Read the model definition and answer for the solid it produces. Units are mm, in the model's axes. Face numbers are marked on the shaded views. A direction names the side the tool comes from. Give positions to 0.01 mm unless a question says otherwise; leave off trailing zeros. Order: outer loops, then holes, each group sorted by start corner. A loop starts at its lowest first (then second) coordinate and runs counter-clockwise, first axis right, second up.
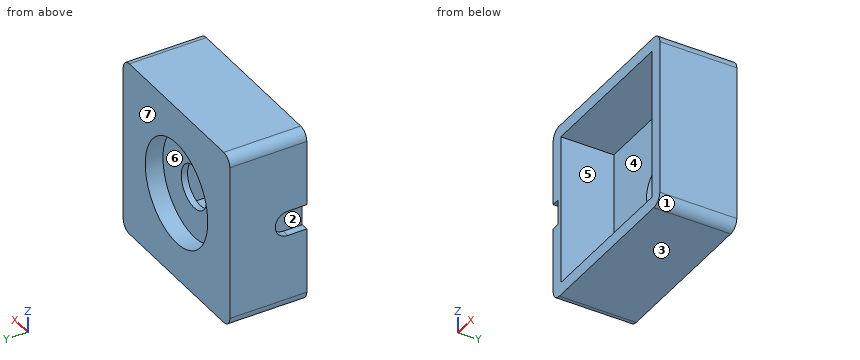
```python
from build123d import *

# Parameters (mm, degrees)
SKETCH_1_W          = 140
SKETCH_1_H          = 140
SKETCH_1_R          = 41
EXTRUDE_1_DEPTH     = 14
SKETCH_3_W          = 140
SKETCH_3_H          = 140
SKETCH_3_R          = 17
EXTRUDE_2_DEPTH     = 5
SKETCH_4_W          = 140
SKETCH_4_H          = 140
SKETCH_4_W_2        = 120
SKETCH_4_H_2        = 120
EXTRUDE_3_DEPTH     = 42
FILLET_3_R          = 8
CUT_EXTRUDE_1_DEPTH = 6


with BuildPart() as part:
    # 草图1 → 凸台-拉伸1 (new body)
    with BuildSketch(Plane(origin=(0, 0, 0), x_dir=(1, 0, 0), z_dir=(0, 1, 0))):
        Rectangle(SKETCH_1_W, SKETCH_1_H)
        with Locations(Location((0, 0, 0), (0, 0, 270))):
            Circle(SKETCH_1_R, mode=Mode.SUBTRACT)
    extrude(amount=EXTRUDE_1_DEPTH)

    # 草图3 → 凸台-拉伸2 (add)
    with BuildSketch(Plane.XZ):
        Rectangle(SKETCH_3_W, SKETCH_3_H)
        with Locations(Location((0, 0, 0), (0, 0, 270))):
            Circle(SKETCH_3_R, mode=Mode.SUBTRACT)
    extrude(amount=EXTRUDE_2_DEPTH)

    # 草图4 → 凸台-拉伸3 (add)
    with BuildSketch(Plane.XZ.offset(5)):
        Rectangle(SKETCH_4_W, SKETCH_4_H)
        Rectangle(SKETCH_4_W_2, SKETCH_4_H_2, mode=Mode.SUBTRACT)
    extrude(amount=EXTRUDE_3_DEPTH)

    # 圆角3
    fillet_3_edges = [part.edges().sort_by_distance(p)[0] for p in [
        (70, -16.5, 70),
        (-70, -16.5, 70),
        (-70, -16.5, -70),
        (70, -16.5, -70),
    ]]
    fillet(fillet_3_edges, radius=FILLET_3_R)

    # 草图5 → 切除-拉伸1 (cut)
    with BuildSketch(Plane.ZY.offset(70)):
        with BuildLine():
            Line((-10, -32), (-10, -47))
            Line((-10, -47), (10, -47))
            Line((10, -47), (10, -32))
            ThreePointArc((10, -32), (0, -22), (-10, -32))
        make_face()
    extrude(amount=-CUT_EXTRUDE_1_DEPTH, mode=Mode.SUBTRACT)


solid = part.part
```
1) The part is cut by section A-A on x = 0. Determine the outline of the cut face in (y, z), and give its area (3 significant figures).
Final values:
outline: (-47, -70) - (14, -70) - (14, -41) - (0, -41) - (0, -17) - (-5, -17) - (-5, -60) - (-47, -60) - close; (-47, 60) - (-5, 60) - (-5, 17) - (0, 17) - (0, 41) - (14, 41) - (14, 70) - (-47, 70) - close
area: 2,180 mm2
2) The part is cut by section C-C on z = 0. Determine the outline of the cut face in (x, y).
Final values:
outline: (-70, -22) - (-64, -22) - (-64, -47) - (-60, -47) - (-60, -5) - (-17, -5) - (-17, 0) - (-41, 0) - (-41, 14) - (-70, 14) - close; (17, -5) - (60, -5) - (60, -47) - (70, -47) - (70, 14) - (41, 14) - (41, 0) - (17, 0) - close
3) Consider L1, parallel to X at y = -28, z = 27; L2, parallel to X at y = 10, z = 0. Determine where each line is inside the solid, lowest interval first.
Final values:
L1: x = -70 to -60, 60 to 70
L2: x = -70 to -41, 41 to 70
4) For a pull along X with two mould halves and no side action, classify the marked faces 1, 2, 3 and 4 as released by +X, released by -X, zero draft, split by the parting line, or undercut.
Final values:
face 1: released by +X
face 2: released by -X
face 3: zero draft
face 4: undercut
5) The part is cut by section B-B on y = -15. Determine the outline of the cut face in (x, z), and give its area (3 significant figures).
Final values:
outline: (-70, -62) arc R8 ccw to (-62, -70) - (62, -70) arc R8 ccw to (70, -62) - (70, 62) arc R8 ccw to (62, 70) - (-62, 70) arc R8 ccw to (-70, 62) - close; hole (-60, -60) - (60, -60) - (60, 60) - (-60, 60) - close
area: 5,150 mm2
6) Given pin 1 (1 mm diameter, centred on x = 37.5, z = 34, fed in from -Y); pin 2 (5 mm diameter, centred on x = -68, y = -41.5, fed in from +Z); pin 3 (1 mm diameter, centred on x = 40, z = -2.5, fed in from +Y), each flat-ended and moving along its own axis, determine where each tip first touches the part or whether it passes through.
Final values:
pin 1: stops at y = -5
pin 2: stops at z = 69.19
pin 3: stops at y = 0
7) The part is cut by section D-D on z = -58. Determine the outline of the cut face in (x, y), and give its area (3 significant figures).
Final values:
outline: (-70, -47) - (-60, -47) - (-60, -5) - (60, -5) - (60, -47) - (70, -47) - (70, 14) - (-70, 14) - close
area: 3,500 mm2
8) A tool of negligible diameter and unlimited length cuts with its end or side. For the marked faces 5, 6 and 7, from which of +Z, -Z, +X, -X, +Y, -Y can it reach the whole face along a straight path? Write none if from no direction.
Final values:
face 5: -Y
face 6: +Y
face 7: +Z, -Z, +X, -X, +Y
